Verification items for this drawing (mm, ordinates from the low corner). Give positions to 0.01 mm unless a question says otherwise; leave off trailing zeros. Order: outer loops, then holes, each group sorted by start corner. A loop starts at its lowest first (then second) coordinate and runs counter-clockwise, first axis right, second up. Notation, with made-up numbers: (66.25, 88.25) -> (78.25, 88.25) arc R14 ccw to (78.25, 113.25) -> close; hole circle Ø3 at (87, 89). An arc over 180 degrees is marked (long way). One line per question, with ' | ' between items.
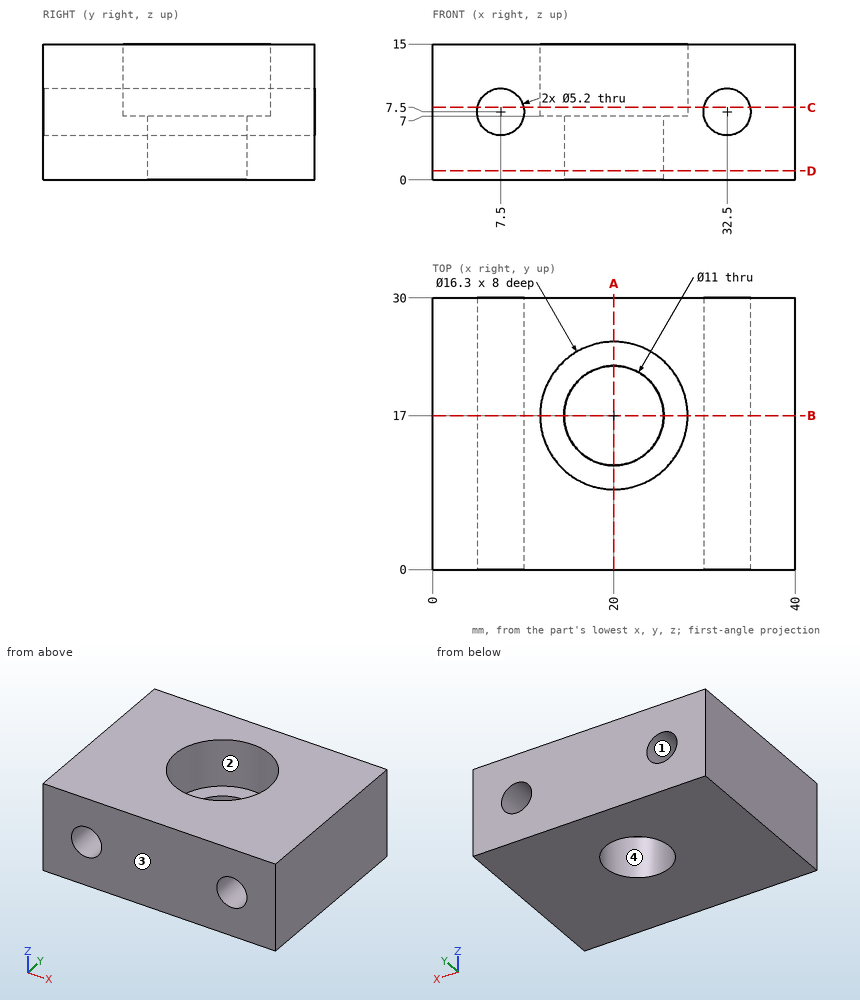
Q1. Section check D-D (z = 1). Enter the section's corners in (x, y).
Result sheet:
outline: (0, 0) -> (40, 0) -> (40, 30) -> (0, 30) -> close; hole circle Ø11 at (20, 17)
Q2. Section check B-B (y = 17). Enter the section's corners in (x, z).
Result sheet:
outline: (0, 0) -> (14.5, 0) -> (14.5, 7) -> (11.85, 7) -> (11.85, 15) -> (0, 15) -> close; (25.5, 0) -> (40, 0) -> (40, 15) -> (28.15, 15) -> (28.15, 7) -> (25.5, 7) -> close; hole circle Ø5.2 at (7.5, 7.5); hole circle Ø5.2 at (32.5, 7.5)
Q3. Section check A-A (x = 20). Enter the section's corners in (y, z).
Result sheet:
outline: (0, 0) -> (11.5, 0) -> (11.5, 7) -> (8.85, 7) -> (8.85, 15) -> (0, 15) -> close; (22.5, 0) -> (30, 0) -> (30, 15) -> (25.15, 15) -> (25.15, 7) -> (22.5, 7) -> close
Q4. Mould release check, pull along Y, two halves, no side actions. Record for the marked faces 1, 2, 3 and 4: pulls with the +Y half, pulls with the -Y half, needs draft (parallel to the pull), parting line crosses it, or undercut.
Result sheet:
face 1: needs draft | face 2: undercut | face 3: pulls with the -Y half | face 4: undercut
Q5. Depth check by flat-ended pin: pin 1 Ø4 at (y, z) = (15.5, 12) entering from -X; pin 2 Ø4 at (x, z) = (32.5, 7.5) entering from -Y; pin 3 Ø8 at (x, y) = (18, 18) entering from +Z. Enter the tip coordinate at first touch or a pass-through.
Result sheet:
pin 1: stops at x = 0 | pin 2: passes through | pin 3: stops at z = 7
Q6. Section check C-C (z = 8). Enter the section's corners in (x, y), and give its area (3 significant figures).
Result sheet:
outline: (0, 0) -> (4.95, 0) -> (4.95, 30) -> (0, 30) -> close; (10.05, 0) -> (29.95, 0) -> (29.95, 30) -> (10.05, 30) -> close; (35.05, 0) -> (40, 0) -> (40, 30) -> (35.05, 30) -> close; hole circle Ø16.3 at (20, 17) | area: 685 mm2
Q7. Thickness scan on line 1 (Z direction, x = 7.5, y = 22.75); line 2 (X direction, y = 17, z = 2); line 3 (X direction, y = 25.5, z = 9). Record the ranges inside material, lowest first.
Result sheet:
line 1: z = 0 to 4.9, 10.1 to 15 | line 2: x = 0 to 14.5, 25.5 to 40 | line 3: x = 0 to 5.38, 9.62 to 30.38, 34.62 to 40
